Geometry: final body of the model. Coordinates: model frame, mm. A direction names the side the tool comes from. Coordinates: 2 decimals unless noted, no trailing zeros. Write each loop counter-clockwise with the first axis right and the second up, starting at its lowest first coordinate (ties: lowest second). Pieces come first, ordered by that corner, then holes.
from build123d import *

# Parameters (mm, degrees)
SKETCH1_W                = 120
SKETCH1_H                = 95
SKETCH1_W_2              = 80
SKETCH1_H_2              = 55
BOSS_EXTRUDE1_DEPTH      = 156
BOSS_EXTRUDE1_DEPTH_BACK = 574
CUT_EXTRUDE1_DEPTH       = 550
CUT_EXTRUDE2_DEPTH       = 20


with BuildPart() as part:
    # Sketch1 → Boss-Extrude1 (new body, two sides)
    with BuildSketch(Plane.XY) as boss_extrude1_sk:
        with Locations((0, 212.5)):
            Rectangle(SKETCH1_W, SKETCH1_H)
        with Locations((0, 212.5)):
            Rectangle(SKETCH1_W_2, SKETCH1_H_2, mode=Mode.SUBTRACT)
    extrude(amount=BOSS_EXTRUDE1_DEPTH)
    extrude(boss_extrude1_sk.sketch, amount=-BOSS_EXTRUDE1_DEPTH_BACK)

    # Sketch2 → Cut-Extrude1 (cut)
    with BuildSketch(Plane(origin=(0, 0, -574), x_dir=(-1, 0, 0), z_dir=(0, 0, -1))):
        Polygon((-40, 165), (-30, 180), (-60, 180), (-60, 165), align=None)
        Polygon((30, 180), (60, 180), (60, 165), (40, 165), align=None)
    extrude(amount=-CUT_EXTRUDE1_DEPTH, mode=Mode.SUBTRACT)

    # Sketch3 → Cut-Extrude2 (cut)
    with BuildSketch(Plane.XZ.offset(-165)):
        with BuildLine():
            Line((-15.640352243, -495.413950444), (-15.640352243, -159.146377226))
            ThreePointArc((-15.640352243, -159.146377226), (0, -143.506024984), (15.640352243, -159.146377226))
            Line((15.640352243, -159.146377226), (15.640352243, -495.413950444))
            ThreePointArc((15.640352243, -495.413950444), (0, -511.054302687), (-15.640352243, -495.413950444))
        make_face()
    extrude(amount=-CUT_EXTRUDE2_DEPTH, mode=Mode.SUBTRACT)


solid = part.part
Item 1: Set-up query: faces 1 (the flat face through (17, 185, -204)), 2 (the flat face through (-1, 260, -204)), 3 (the flat face through (15.64, 175, -325)), 4 (the flat face through (-45, 180, -303)), 5 (the flat face through (49, 173, -24)). Return all of +Z, -Z, +X, -X, +Y, -Y with unobstructed straight access to the full face (end or side cutting, diameter ignored); none if empty.
Derived:
face 1: +Z, -Z
face 2: +Z, -Z, +X, -X, +Y
face 3: -Y
face 4: -Z, -X
face 5: -Z, +X
Item 2: Pin query (flat end, axial travel): pin 1 (10 mm diameter, centred on y = 172, z = -330.5, fed in from -X); pin 2 (1 mm diameter, centred on y = 178.5, z = -31, fed in from +X); pin 3 (22 mm diameter, centred on y = 173, z = -351, fed in from +X); pin 4 (5 mm diameter, centred on x = -46.5, z = -63, fed in from -Y). Return the tip coordinate at first contact, or that it passes through.
Derived:
pin 1: stops at x = -38.67
pin 2: stops at x = 31.33
pin 3: stops at x = 60
pin 4: stops at y = 180
Item 3: Pull-direction query (Y, two-part tool) for faces 6 (the flat face through (45, 180, -303)), 7 (the flat face through (60, 212, -204)), 8 (the flat face through (-1, 165, -123)), 9 (the flat face through (35.07, 172.395, -302.85)); classes: released by +Y, released by -Y, zero draft, split by the parting line, or undercut.
Derived:
face 6: undercut
face 7: zero draft
face 8: released by -Y
face 9: undercut
Item 4: Material intervals for probe 1 along X at (y, z) = (209.5, 65); probe 2 along Y at (x, z) = (-15, 1); probe 3 along X at (y, z) = (180.5, -428.5), sorted ascending.
Derived:
probe 1: x = -60 to -40, 40 to 60
probe 2: y = 165 to 185, 240 to 260
probe 3: x = -60 to -15.64, 15.64 to 60
Item 5: Section B-B, the plane y = 218.5. Output: boundary loops of the cut face in (x, z), plus the area to 3 significant figures.
Derived:
outline: (-60, -574) - (-40, -574) - (-40, 156) - (-60, 156) - close; (40, -574) - (60, -574) - (60, 156) - (40, 156) - close
area: 29,200 mm2
Item 6: Section D-D, the plane z = -389.5. Output: boundary loops of the cut face in (x, y), plus the area to 3 significant figures.
Derived:
outline: (-60, 180) - (-30, 180) - (-40, 165) - (-15.64, 165) - (-15.64, 185) - (-40, 185) - (-40, 240) - (40, 240) - (40, 185) - (15.64, 185) - (15.64, 165) - (40, 165) - (30, 180) - (60, 180) - (60, 260) - (-60, 260) - close
area: 5,620 mm2
Item 7: Section A-A, the plane x = 0. Output: boundary loops of the cut face in (y, z).
Derived:
outline: (165, -574) - (185, -574) - (185, -511.05) - (165, -511.05) - close; (165, -143.51) - (185, -143.51) - (185, 156) - (165, 156) - close; (240, -574) - (260, -574) - (260, 156) - (240, 156) - close
Item 8: Section C-C, the plane z = 101. Output: boundary loops of the cut face in (x, y), plus the area to 3 significant figures.
Derived:
outline: (-60, 165) - (60, 165) - (60, 260) - (-60, 260) - close; hole (-40, 185) - (40, 185) - (40, 240) - (-40, 240) - close
area: 7,000 mm2
